Source: CAD feature listing. Evaluate the final solid. Frame: model axes, mm. A direction names the side the tool comes from. Round coordinates to 2 decimals unless told otherwise and drop trailing zeros. Loops run counter-clockwise (first coordinate to the right, second up) from the corner with the lowest first, then second, coordinate; pieces in that order, holes last. Notation, with made-up numbers: M -17,5.25 L 27,5.25 A10 ccw 27,16.25 Z; hole C 24,16 d7. An arc over 180 degrees is marked long. Answer as a JSON object with one key per item and string values.
Autodesk Inventor part; units mm, degrees
ref_plane "YZ Plane" through (0, 0, 0) normal (1, 0, 0) x (0, 1, 0)
ref_plane "XZ Plane" through (0, 0, 0) normal (0, 1, 0) x (-1, 0, 0)
ref_plane "XY Plane" through (0, 0, 0) normal (0, 0, 1) x (1, 0, 0)
sketch "Sketch1" plane through (0, 0, 0) normal (0, 0, 1) x (1, 0, 0)
  line L0 (-30, 0) -> (30, 0) construction
  circle A0 centre (-30, 0) radius 4
  circle A1 centre (30, 0) radius 4
  line L1 (-30, 0) -> (30, 0) construction
  line L2 (-30, -7) -> (30, -7)
  line L3 (30, 7) -> (-30, 7)
  arc A2 (-30, 7) -> (-30, -7) centre (-30, 0) ccw
  arc A3 (30, -7) -> (30, 7) centre (30, 0) ccw
  point P0 (0, 0)
  point P1 (0, 0)
  point P2 (0, 0)
  dimension "d0" = 60
  dimension "d1" = 8
  dimension "d2" = 7
extrude "Extrusion1" add sketch "Sketch1" along normal blind 25
sketch "Sketch2" plane through (-30, -7, 0) normal (0, -1, 0) x (1, 0, 0)
  line L0 (0, 0) -> (60, 0) construction
  line L1 (60, 0) -> (60, 25) construction
  line L2 (0, 25) -> (60, 25) construction
  line L3 (0, 0) -> (0, 25) construction
  line L4 (30, 25) -> (30, 0) construction
  circle A0 centre (30, 12.5) radius 9.375
  dimension "d5" = 18.75
extrude "Extrusion2" cut sketch "Sketch2" against normal through all
sketch "Sketch3" plane through (-30, 7, 0) normal (0, 1, 0) x (1, 0, 0)
  circle A0 centre (30, -12.5) radius 9.375
  circle A1 centre (30, -12.5) radius 12.5
  line L0 (60, -25) -> (0, -25)
  point P0 (30, 0)
extrude "Extrusion3" add sketch "Sketch3" along normal blind 10
sketch "Sketch4" plane through (0, 0, 25) normal (0, 0, 1) x (1, 0, 0)
  circle A0 centre (0, 0) radius 3
  dimension "d10" = 6
extrude "Extrusion4" cut sketch "Sketch4" against normal up to next
properties part number "reed switch holder"
Item 1: Access query for faces 1 (the cylindrical face through (5.77, 11.93, 1.41)), 2 (the cylindrical face through (-2.032, 4.832, 3.348)). Directions: +Z, -Z, +X, -X, +Y, -Y. A direction counts if a zero-diameter tool reaches every point of the face in a straight line with its end or side. Return the directions, or none.
Answer sheet:
{"face 1": "+Y", "face 2": "+Y, -Y"}
Item 2: Section D-D on x = 18. Return the cut outline in (y, z), then the cut area to 3 significant figures.
Answer sheet:
{"outline": "M -7,0 L 7,0 L 7,25 L -7,25 Z", "area": "350 mm²"}
Item 3: Pull-direction query (Y, two-part tool) for faces 3 (the cylindrical face through (-33.2, 2.4, 12.3)), 4 (the cylindrical face through (-0.65, -2.93, 23.22)), 5 (the flat face through (2, 17, 3)), 6 (the flat face through (-1, 3, 25)); classes: pulls with the +Y half, pulls with the -Y half, needs draft (parallel to the pull), parting line crosses it, or undercut.
Answer sheet:
{"face 3": "undercut", "face 4": "undercut", "face 5": "pulls with the +Y half", "face 6": "needs draft"}
Item 4: Line query: probe 1 along Z at (x, y) = (0, 10) (3 decimals); probe 2 along Y at (x, z) = (-30, 16.25); probe 3 along X at (y, z) = (-1.5, 20.5). Output: solid intervals per line, ascending. Write a range as from..to.
Answer sheet:
{"probe 1": "z = 0..3.125, 21.875..25", "probe 2": "y = -7..-4, 4..7", "probe 3": "x = -36.84..-33.71, -26.29..-4.89, 4.89..26.29, 33.71..36.84"}
Item 5: Section A-A on x = 6. Return the cut outline in (y, z), then the cut area to 3 significant figures.
Answer sheet:
{"outline": "M -7,0 L 7,0 L 7,1.53 L 17,1.53 L 17,5.3 L -7,5.3 Z; M -7,19.7 L 17,19.7 L 17,23.47 L 7,23.47 L 7,25 L -7,25 Z", "area": "224 mm²"}
Item 6: Section B-B on y = 1.5. Return the cut outline in (x, z) (3 decimals).
Answer sheet:
{"outline": "M -36.837,0 L -33.708,0 L -33.708,25 L -36.837,25 Z; M -26.292,0 L 26.292,0 L 26.292,25 L 2.598,25 L 2.598,21.508 A9.375 cw long -2.598,21.508 L -2.598,25 L -26.292,25 Z; M 33.708,0 L 36.837,0 L 36.837,25 L 33.708,25 Z"}
Item 7: Section C-C on y = 8.5. Return the cut outline in (x, z) (3 decimals), then the cut area to 3 significant figures.
Answer sheet:
{"outline": "C 0,12.5 d25; hole C 0,12.5 d18.75", "area": "215 mm²"}
Item 8: Contact query for flat-ended pins moving along their axis: pin 1 Ø8 at (y, z) = (11.5, 13) entering from +X; pin 2 Ø13 at (x, y) = (30, 0) entering from -Z; pin 3 Ø6 at (y, z) = (8, 5.5) entering from +X; pin 4 Ø1 at (y, z) = (-1.5, 16) entering from -X. Output: stop coordinate, or through.
Answer sheet:
{"pin 1": "stops at x = 12.5", "pin 2": "stops at z = 0", "pin 3": "stops at x = 34.9", "pin 4": "stops at x = -36.93"}
